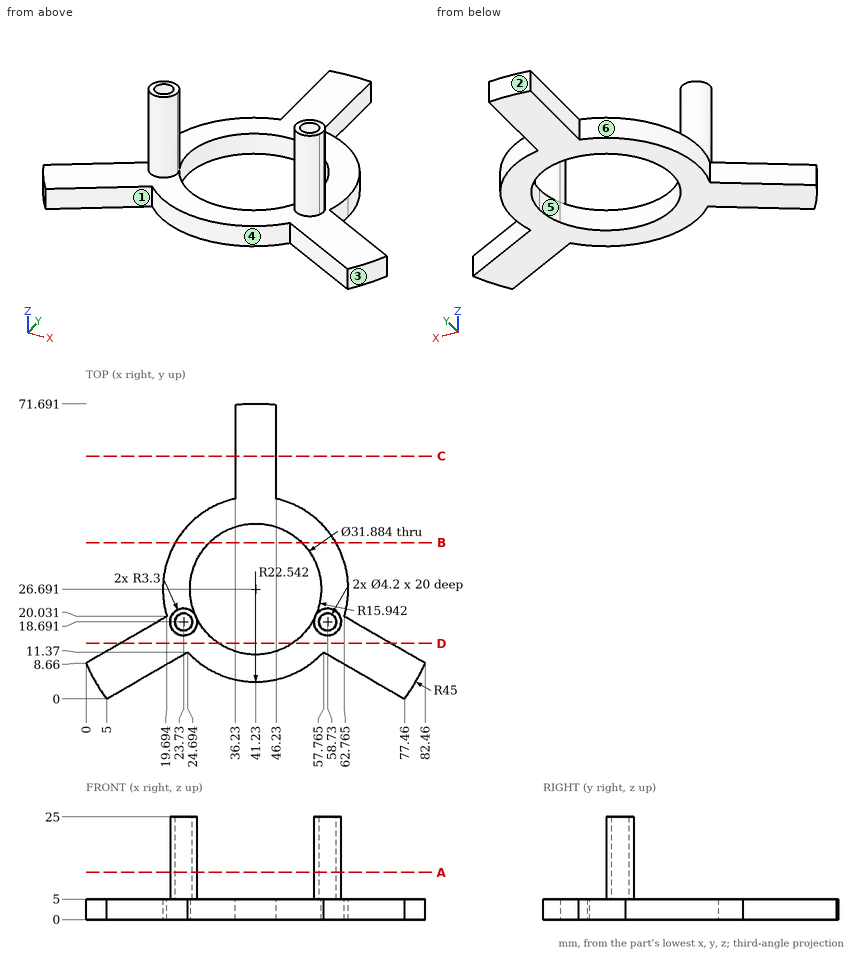
Here's the drawing with two shaded views (mm, measured from the low corner). I have some questions. A direction names the side the tool comes from. Give positions to 0.01 mm unless a question says otherwise; leave off trailing zeros. Order: outer loops, then holes, each group sorted by start corner. A loop starts at its lowest first (then second) coordinate and runs counter-clockwise, first axis right, second up. Notation, with made-up numbers: (3, 7) -> (37, 7) arc R33 ccw to (37, 38) -> close; hole circle Ø7 at (35, 1). An arc over 180 degrees is marked (long way). Use a Markdown table: item, result. Add a question column.
Item 1: If we mould it in two halves opening along X, with no side actions, what happens to the marked faces 3, 4, 5 and 6? For each: pulls with the +X half, pulls with the -X half, needs draft (parallel to the pull), parting line crosses it, or undercut.
Item 2: Imagine slicing it at D-D on y = 13.5. Please give me the cut outline in (x, z), plus the area to 3 significant figures.
Item 3: Will these pins go through, and if not, where does the flat tip stop? pin 1 (2 mm diameter, centred on x = 59, y = 18, fed in from +Z); pin 2 (5.5 mm diameter, centred on y = 55, z = 2.5, fed in from -X); pin 3 (8 mm diameter, centred on x = 20, z = 4.5, fed in from +Y) (1 decimal).
Item 4: Imagine slicing it at C-C on y = 59. Please give me the cut outline in (x, z), plus the area to 3 significant figures.
Item 5: For the marked faces 1 and 2, which set-ups out of +Z, -Z, +X, -X, +Y, -Y let a thin tool reach every point of the face, with its end or its side?
Item 6: I need wall thicknesses on line 1 (X direction, y = 19.5, z = 21.75); line 2 (Z direction, x = 39.5, y = 9); line 3 (Y direction, x = 25, z = 22) (1 decimal). Which ranges of each line are inside material? Lowest first, please.
Item 7: Imagine slicing it at A-A on z = 11.5. Please give me the cut outline in (x, y).
Item 8: Imagine slicing it at B-B on y = 38. Please give me the cut outline in (x, z) (1 decimal).
Data:
| question | item | result |
|---|---|---|
| 1 | face 3 | pulls with the +X half |
| 1 | face 4 | undercut |
| 1 | face 5 | undercut |
| 1 | face 6 | pulls with the -X half |
| 2 | outline | (8.38, 0) -> (32.28, 0) -> (32.28, 5) -> (8.38, 5) -> close; (50.18, 0) -> (74.08, 0) -> (74.08, 5) -> (50.18, 5) -> close |
| 2 | area | 239 mm² |
| 3 | pin 1 | stops at z = 5 |
| 3 | pin 2 | stops at x = 36.23 |
| 3 | pin 3 | stops at y = 41.2 |
| 4 | outline | (36.23, 0) -> (46.23, 0) -> (46.23, 5) -> (36.23, 5) -> close |
| 4 | area | 50.0 mm² |
| 5 | face 1 | +Z, -Z, -Y |
| 5 | face 2 | +Z, -Z, +Y |
| 6 | line 1 | x = 20.53 to 21.79, 25.67 to 26.93, 55.53 to 56.79, 60.67 to 61.93 |
| 6 | line 2 | z = 0 to 5 |
| 6 | line 3 | y = 15.6 to 17, 20.4 to 21.7 |
| 7 | outline | (26.73, 20.06) arc R3.3 ccw (long way) to (27.03, 18.69) arc R3.3 ccw to start; (61.73, 17.32) arc R3.3 ccw to (62.03, 18.69) arc R3.3 ccw (long way) to start; hole circle Ø4.2 at (23.73, 18.69); hole circle Ø4.2 at (58.73, 18.69) |
| 8 | outline | (21.7, 0) -> (30, 0) -> (30, 5) -> (21.7, 5) -> close; (52.5, 0) -> (60.7, 0) -> (60.7, 5) -> (52.5, 5) -> close |
